Design review of the part built by this model. Coordinates are the model's own, in mm. Coordinates: 2 decimals unless noted, no trailing zeros. Write each loop counter-clockwise with the first axis right and the second up, starting at its lowest first coordinate (ties: lowest second). Pieces come first, ordered by that corner, then holes.
Q1. For probe 1 along X at (y, z) = (0.35, 0); probe 2 along X at (y, z) = (0.65, 2); probe 3 along Z at (x, y) = (1, 0.6), list the stretches that pass through material, from the lowest coordinate up.
Q2. Take a section at A-A (z = 0). Give the boundary of the cut face in (x, y).
Q3. Take a section at B-B (x = 0). Give the boundary of the cut face in (y, z), and give its area (3 significant figures).
Q4. Take a section at C-C (y = 0.4). Give the boundary of the cut face in (x, z).
Q5. Take a section at D-D (x = 14). Give the boundary of the cut face in (y, z).
Q6. Insertion check: pin 1 (6.5 mm diameter, centred on x = -15, z = 0, fed in from +Y). The pin has a flat end and moves straight along its axis. Give the tip position at first contact, or say it passes through.
Q7. Mouldability with a two-part tool opening along X and no side actions: class faces 1 (the cylindrical face through (0.121, 0.426, 12.253)), 2 (the cylindrical face through (-8.366, 0.426, 20.178)), 3 (the flat face through (-5, 0, 9)) as pulls with the +X half, pulls with the -X half, needs draft (parallel to the pull), parting line crosses it, or undercut.
```python
from build123d import *

# Parameters (mm, degrees)
SKETCH1_R           = 21.844
SKETCH1_R_2         = 2.75
BOSS_EXTRUDE1_DEPTH = 0.8636
SKETCH2_R           = 9.652
CUT_EXTRUDE1_DEPTH  = 0.8636


with BuildPart() as part:
    # Sketch1 → Boss-Extrude1 (new body)
    with BuildSketch(Plane(origin=(0, 0, 0), x_dir=(1, 0, 0), z_dir=(0, 1, 0))):
        with Locations(Location((0, 0, 0), (0, 0, 270))):
            Circle(SKETCH1_R)
        with Locations(Location((0, 15, 0), (0, 0, 270))):
            Circle(SKETCH1_R_2, mode=Mode.SUBTRACT)
        with Locations(Location((15, 0, 0), (0, 0, 270))):
            Circle(SKETCH1_R_2, mode=Mode.SUBTRACT)
        with Locations(Location((0, -15, 0), (0, 0, 270))):
            Circle(SKETCH1_R_2, mode=Mode.SUBTRACT)
        with Locations(Location((-15, 0, 0), (0, 0, 270))):
            Circle(SKETCH1_R_2, mode=Mode.SUBTRACT)
    extrude(amount=BOSS_EXTRUDE1_DEPTH)

    # Sketch2 → Cut-Extrude1 (cut)
    with BuildSketch(Plane.XZ):
        with Locations(Location((0, 0, 0), (0, 0, 270))):
            Circle(SKETCH2_R)
    extrude(amount=-CUT_EXTRUDE1_DEPTH, mode=Mode.SUBTRACT)


solid = part.part
```
Response:
1. probe 1: x = -21.84 to -17.75, -12.25 to -9.65, 9.65 to 12.25, 17.75 to 21.84
1. probe 2: x = -21.75 to -16.89, -13.11 to -9.44, 9.44 to 13.11, 16.89 to 21.75
1. probe 3: z = -21.82 to -17.56, -12.44 to -9.6, 9.6 to 12.44, 17.56 to 21.82
2. outline: (-21.84, 0) - (-17.75, 0) - (-17.75, 0.86) - (-21.84, 0.86) - close; (-12.25, 0) - (-9.65, 0) - (-9.65, 0.86) - (-12.25, 0.86) - close; (9.65, 0) - (12.25, 0) - (12.25, 0.86) - (9.65, 0.86) - close; (17.75, 0) - (21.84, 0) - (21.84, 0.86) - (17.75, 0.86) - close
3. outline: (0, -21.84) - (0.86, -21.84) - (0.86, -17.75) - (0, -17.75) - close; (0, -12.25) - (0.86, -12.25) - (0.86, -9.65) - (0, -9.65) - close; (0, 9.65) - (0.86, 9.65) - (0.86, 12.25) - (0, 12.25) - close; (0, 17.75) - (0.86, 17.75) - (0.86, 21.84) - (0, 21.84) - close
3. area: 11.6 mm2
4. outline: circle Ø43.69 at (0, 0); hole circle Ø5.5 at (-15, 0); hole circle Ø19.3 at (0, 0); hole circle Ø5.5 at (0, -15); hole circle Ø5.5 at (0, 15); hole circle Ø5.5 at (15, 0)
5. outline: (0, -16.77) - (0.86, -16.77) - (0.86, -2.56) - (0, -2.56) - close; (0, 2.56) - (0.86, 2.56) - (0.86, 16.77) - (0, 16.77) - close
6. pin 1: stops at y = 0.86
7. face 1: undercut
7. face 2: parting line crosses it
7. face 3: needs draft
